```python
from build123d import *
from build123d.topology import SkipClean

# Parameters (mm, degrees)
EXTRUSION1_DEPTH = 36.869499995
THREAD6_D        = 5.25
THREAD6_DEPTH    = 20
THREAD6_TIP      = 1.577259125
THREAD10_D       = 5.25
THREAD10_DEPTH   = 17
SKETCH6_W        = 48
SKETCH6_H        = 36.869499995
SKETCH6_R        = 2.625
EXTRUSION2_DEPTH = 1.869499995


with BuildPart() as part:
    # Sketch1 → Extrusion1 (new body)
    with BuildSketch(Plane.XY):
        with BuildLine():
            Line((-24, 20), (24, 20))
            Line((24, 20), (24, -20))
            Line((24, -20), (8.5, -20))
            Line((8.5, -20), (8.5, -11.187157816))
            ThreePointArc((8.5, -11.187157816), (0, 14.05), (-8.5, -11.187157816))
            Line((-8.5, -11.187157816), (-8.5, -20))
            Line((-8.5, -20), (-24, -20))
            Line((-24, -20), (-24, 20))
        make_face()
    extrude(amount=EXTRUSION1_DEPTH)

    # Thread6
    with Locations(Plane.XY.offset(36.869499995)):
        with Locations((-19, 0), (-13.435028843, -13.435028843), (-13.435028843, 13.435028843), (13.435028843, 13.435028843), (19, 0), (13.435028843, -13.435028843)):
            Hole(THREAD6_D / 2, depth=THREAD6_DEPTH)
            with Locations((0, 0, -(THREAD6_DEPTH + THREAD6_TIP / 2))):  # 118° drill point
                Cone(0, THREAD6_D / 2, THREAD6_TIP, mode=Mode.SUBTRACT)

    # Thread10
    with Locations(Plane(origin=(0, 20, 0), x_dir=(1, 0, 0), z_dir=(0, 1, 0))):
        with Locations((-19, -6.5), (19, -6.5), (-19, -28.5), (19, -28.5)):
            Hole(THREAD10_D / 2, depth=THREAD10_DEPTH)

    # Sketch6 → Extrusion2 (add)
    with SkipClean():  # the faces are left unmerged after this step: merging them gives an invalid solid
        with BuildSketch(Plane(origin=(0, 20, 0), x_dir=(-1, 0, 0), z_dir=(0, 1, 0))):
            with Locations((0, 18.434749998)):
                Rectangle(SKETCH6_W, SKETCH6_H)
            with Locations(Location((19, 28.5, 0), (0, 0, 90))):
                Circle(SKETCH6_R, mode=Mode.SUBTRACT)
            with Locations(Location((19, 6.5, 0), (0, 0, 90))):
                Circle(SKETCH6_R, mode=Mode.SUBTRACT)
            with Locations(Location((-19, 6.5, 0), (0, 0, 90))):
                Circle(SKETCH6_R, mode=Mode.SUBTRACT)
            with Locations(Location((-19, 28.5, 0), (0, 0, 90))):
                Circle(SKETCH6_R, mode=Mode.SUBTRACT)
        extrude(amount=EXTRUSION2_DEPTH)


solid = part.part
```
The model under review builds one solid part; all positions refer to its coordinate system, in mm. A direction names the side the tool comes from. Round coordinates to 2 decimals unless told otherwise and drop trailing zeros. Order: outer loops, then holes, each group sorted by start corner. A loop starts at its lowest first (then second) coordinate and runs counter-clockwise, first axis right, second up.
Item 1: To check wall thickness, follow probe 1 along Z at (x, y) = (19, 20.8) (1 decimal); probe 2 along Y at (x, z) = (19, 27) (3 decimals); probe 3 along Z at (x, y) = (17, 9.5). State the ranges of each line that lie inside material, in increasing order.
Working result:
probe 1: z = 0 to 3.9, 9.1 to 25.9, 31.1 to 36.9
probe 2: y = -20 to -2.625, 2.625 to 3
probe 3: z = 0 to 4.8, 8.2 to 26.8, 30.2 to 36.87
Item 2: For pin 1 (3 mm diameter, centred on x = -13, y = -6.5, fed in from -Z); pin 2 (2 mm diameter, centred on x = -5.5, y = 11.5, fed in from -Z); pin 3 (4 mm diameter, centred on x = -19, y = 0, fed in from +Z), all flat-tipped, find the tip position at first contact; note any pin that passes through.
Working result:
pin 1: stops at z = 0
pin 2: passes through
pin 3: stops at z = 16.49
Item 3: Machinability: for faces 5 (the cylindrical face through (12.22, -15.76, 26.73)), 6 (the flat face through (-8.5, -16, 18)), 7 (the cylindrical face through (0.49, 14.04, 18.18)), 8 (the flat face through (19, 3, 28)), which of the approach directions +Z, -Z, +X, -X, +Y, -Y give a long, thin tool a straight path to every point of the face, cutting with its end or side? Answer none if there is none.
Working result:
face 5: +Z
face 6: +Z, -Z, -Y
face 7: +Z, -Z
face 8: +Y
Item 4: Draft analysis for pull direction Z (two halves, no side actions). For faces 1 (the flat face through (16, -20, 18)), 2 (the flat face through (-19, 3, 6)), 3 (the conical face through (-19.46, 0.02, 15.57)), 4 (the flat face through (19, 3, 6)), state which applies: released by +Z, released by -Z, zero draft, split by the parting line, or undercut.
Working result:
face 1: zero draft
face 2: undercut
face 3: released by +Z
face 4: undercut
Item 5: Add section D-D, the plane y = -6. State the section outline as (x, z) points, and give its area (3 significant figures).
Working result:
outline: (-24, 0) - (-12.7, 0) - (-12.7, 36.87) - (-24, 36.87) - close; (12.7, 0) - (24, 0) - (24, 36.87) - (12.7, 36.87) - close
area: 833 mm2
Item 6: Add section B-B, the plane z = 3. State the section outline as (x, y) points.
Working result:
outline: (-24, -20) - (-8.5, -20) - (-8.5, -11.19) arc R14.05 cw (long way) to (8.5, -11.19) - (8.5, -20) - (24, -20) - (24, 21.87) - (-24, 21.87) - close
Item 7: Add section A-A, the plane y = 4. Count the separate pieces of the cut face and the enclosed holes in it, and give its area (3 significant figures).
Working result:
separate pieces: 2
enclosed holes: 4
area: 690 mm2
